Here's how the part is built. I have some questions about the finished solid (model axes, mm). A direction names the side the tool comes from. Coordinates: 2 decimals unless noted, no trailing zeros. Write each loop counter-clockwise with the first axis right and the second up, starting at its lowest first coordinate (ties: lowest second). Pieces come first, ordered by that corner, then holes. Notation, with made-up numbers: M -34,31 L -17,31 A32 cw -17,69 Z; hole C 89,53.5 d7. An arc over 180 degrees is marked long. Use a Markdown table: item, result.
Autodesk Inventor part; units mm, degrees
ref_plane "YZ Plane" through (0, 0, 0) normal (1, 0, 0) x (0, 1, 0)
ref_plane "XZ Plane" through (0, 0, 0) normal (0, 1, 0) x (-1, 0, 0)
ref_plane "XY Plane" through (0, 0, 0) normal (0, 0, 1) x (1, 0, 0)
sketch "Skizze1" plane through (0, 0, 0) normal (1, 0, 0) x (0, 1, 0)
  line L0 (0, -102) -> (0, 17)
  line L1 (-6.4, 0) -> (38.4, 0)
  line L2 (0, 0) -> (32, 0)
  line L3 (32, 0) -> (32, -85)
  line L4 (32, -85) -> (0, -85)
  line L5 (0, -85) -> (0, 0)
  line L6 (0, 0) -> (10, 0)
  line L7 (10, 0) -> (22, 0)
  line L8 (22, 0) -> (22, -22)
  line L9 (10, -22) -> (10, 0)
  line L10 (10, -85) -> (22.1, -85)
  line L11 (22.1, -85) -> (22.1, -63)
  line L12 (10, -63) -> (10, -85)
  line L13 (22, -22) -> (10, -22)
  line L14 (10, -63) -> (22.1, -63)
  line L15 (32, -2.5) -> (22, -2.5)
  line L16 (10, -2.5) -> (0, -2.5)
  line L17 (32, -85) -> (32, -82.5)
  line L18 (32, -82.5) -> (22.1, -82.5)
  line L19 (10, -82.5) -> (0, -82.5)
  point P0 (16, -42.5)
  dimension "d0" = 32
  dimension "d1" = 85
  dimension "d2" = 10
  dimension "d4" = 22
  dimension "d5" = 12
  dimension "d8" = 2.5
extrude "Extrusion2" add sketch "Skizze1" along normal blind 20 contours L0 L19 L12 L4 | L0 L16 L9 L13 L8 L15 L3 L18 L11 L14 L12 L19 | L0 L1 L9 L16 | L11 L18 L3 L4 | L1 L3 L15 L8
chamfer "Fasen5" distance 2.5 angle 45 1 edges at (10, 0, -85) measured on face at (6.6667, 0, -28.3333)
chamfer "Fasen6" distance 2.5 angle 45 1 edges at (10, 32, -85) measured on face at (6.6667, 32, -56.6667)
chamfer "Fasen7" distance 2.5 angle 45 1 edges at (10, 32, 0) measured on face at (13.3333, 32, -55)
chamfer "Fasen8" distance 2.5 angle 45 1 edges at (10, 0, 0) measured on face at (13.3333, 0, -27.5)
hole "Bohrung1" at (0, 16, -42.5) direction (1, 0, 0) diameter 12 end through all
thread "Gewinde1"
sketch "Skizze2" plane through (0, 32, -82.5) normal (0, 1, 0) x (1, 0, 0)
  line L0 (0, 2.5) -> (0, -19.5)
  line L1 (0, 2.5) -> (0, -7.5)
  point P0 (0, -82.5)
  point P1 (10, -7.5)
  point P2 (0, -72.5)
  point P3 (10, -72.047)
hole "Bohrung2" at (10, 32, -75) at (10, 32, -10.453) direction (0, -1, 0) diameter 8 end through all
chamfer "Fasen9" distance 2.5 angle 45 1 edges at (20, 25.75, 0) measured on face at (13.3333, 27, 0)
chamfer "Fasen10" distance 2.5 angle 45 1 edges at (20, 6.25, 0) measured on face at (13.3333, 7.5, 0)
chamfer "Fasen11" distance 2.5 angle 45 1 edges at (20, 25.8, -85) measured on face at (13.3333, 24.5667, -85)
chamfer "Fasen12" distance 2.5 angle 45 1 edges at (20, 6.25, -85) measured on face at (13.3333, 5, -85)
chamfer "Fasen13" distance 2.5 angle 45 1 edges at (0, 25.8, -85) measured on face at (5.8333, 24.5667, -85)
chamfer "Fasen14" distance 2.5 angle 45 1 edges at (0, 6.25, -85) measured on face at (5.8333, 5, -85)
chamfer "Fasen15" distance 2.5 angle 45 1 edges at (0, 25.75, 0) measured on face at (0, 28.6521, -42.2589)
chamfer "Fasen16" distance 2.5 angle 45 1 edges at (0, 6.25, 0) measured on face at (0, 3.3479, -42.7411)
properties part number "Abzieher_Trägeript" material "1.0038 S235JR"
1. We'd pull the mould along Y, two halves only. Please class faces 1 (the face through (18.7, 26, -83.8)), 2 (the face through (5, 22.1, -74)), 3 (the face through (10.1, 1.2, -1.3)): +Y half, -Y half, draft (parallel to the pull), parting line (faces both ways), or undercut.
Answers follow:
| item | result |
|---|---|
| face 1 | draft |
| face 2 | undercut |
| face 3 | -Y half |
2. Suppose I cut it at D-D on y = 7.5. Write out the boundary of the cut face in (x, z).
Answers follow:
| item | result |
|---|---|
| outline | M 0,-82.5 L 2.5,-85 L 17.5,-85 L 20,-82.5 L 20,-2.5 L 17.5,0 L 2.5,0 L 0,-2.5 Z; hole C 10,-75 d8; hole C 10,-10.45 d8 |
3. Suppose I cut it at B-B on z = -42.5. Write out the boundary of the cut face in (x, y), and give its area (3 significant figures).
Answers follow:
| item | result |
|---|---|
| outline | M 0,0 L 20,0 L 20,10 L 0,10 Z; M 0,22 L 20,22 L 20,32 L 0,32 Z |
| area | 400 mm2 |
4. Suppose I cut it at C-C on z = -75. Write out the boundary of the cut face in (x, y), and give its area (3 significant figures).
Answers follow:
| item | result |
|---|---|
| outline | M 0,0 L 6,0 L 6,10 L 0,10 Z; M 0,22.1 L 6,22.1 L 6,32 L 0,32 Z; M 14,0 L 20,0 L 20,10 L 14,10 Z; M 14,22.1 L 20,22.1 L 20,32 L 14,32 Z |
| area | 239 mm2 |
5. Which directions (+Z, -Z, +X, -X, +Y, -Y) give clear straight access to the entire face, cutting with the end or side of a thin tool? Please do faces 4 (the face through (12, 10, -71)), 5 (the face through (14.3, 10, -11.2)), 6 (the face through (10.1, 30.8, -83.7)).
Answers follow:
| item | result |
|---|---|
| face 4 | -Z, +X, -X |
| face 5 | +Z, +X, -X |
| face 6 | -Z, +X, -X, +Y |
6. I need wall thicknesses on probe 1 along Z at (x, y) = (10, 25); probe 2 along Z at (x, y) = (10, 16); probe 3 along Z at (x, y) = (10, 30). Which ranges of each line are inside material? Lowest first, please.
Answers follow:
| item | result |
|---|---|
| probe 1 | z = -85 to -79, -71 to -14.45, -6.45 to 0 |
| probe 2 | z = -63 to -48.5, -36.5 to -22 |
| probe 3 | z = -84.5 to -79, -71 to -14.45, -6.45 to -0.5 |
7. Suppose I cut it at A-A on x = 10. State how many separate pieces and enclosed holes the cut face has, and give its area (4 significant figures).
Answers follow:
| item | result |
|---|---|
| separate pieces | 5 |
| enclosed holes | 1 |
| area | 1,745 mm2 |
